Work out the finished part from the listing and answer in its coordinate system (mm). A direction names the side the tool comes from. Give positions to 0.01 mm unless a question says otherwise; leave off trailing zeros. One line per item, written item: value.
from build123d import *

# Parameters (mm, degrees)
F0_R     = 14
F1_DEPTH = 1.6
F2_R     = 2.25
F3_DEPTH = 2.2


with BuildPart() as f1:
    # F0 (on Top) → F1 (new body)
    with BuildSketch(Plane.XY):
        with BuildLine():
            Line((55.331106, 31.643028), (43.487067, 43.487067))
            Line((43.487067, 43.487067), (31.643028, 55.331106))
            ThreePointArc((31.643028, 55.331106), (16.240585, 49.856732), (0, 48))
            ThreePointArc((0, 48), (-16.240585, 49.856732), (-31.643028, 55.331106))
            Line((-31.643028, 55.331106), (-43.487067, 43.487067))
            Line((-43.487067, 43.487067), (-55.331106, 31.643028))
            ThreePointArc((-55.331106, 31.643028), (-49.856732, 16.240585), (-48, 0))
            ThreePointArc((-48, 0), (-49.856732, -16.240585), (-55.331106, -31.643028))
            Line((-55.331106, -31.643028), (-43.487067, -43.487067))
            Line((-43.487067, -43.487067), (-31.643028, -55.331106))
            ThreePointArc((-31.643028, -55.331106), (-16.240585, -49.856732), (0, -48))
            ThreePointArc((0, -48), (16.240585, -49.856732), (31.643028, -55.331106))
            Line((31.643028, -55.331106), (43.487067, -43.487067))
            Line((43.487067, -43.487067), (55.331106, -31.643028))
            ThreePointArc((55.331106, -31.643028), (49.856732, -16.240585), (48, 0))
            ThreePointArc((48, 0), (49.856732, 16.240585), (55.331106, 31.643028))
        make_face()
        with BuildLine():
            ThreePointArc((-40.092954, -40.092954), (-41.557421, -36.557421), (-40.092954, -33.021887))
            Line((-40.092954, -33.021887), (-32.385491, -25.314423))
            ThreePointArc((-32.385491, -25.314423), (-28.849957, -23.849957), (-25.314423, -25.314423))
            ThreePointArc((-25.314423, -25.314423), (-23.849957, -28.849957), (-25.314423, -32.385491))
            Line((-25.314423, -32.385491), (-33.021887, -40.092954))
            ThreePointArc((-33.021887, -40.092954), (-36.557421, -41.557421), (-40.092954, -40.092954))
        make_face(mode=Mode.SUBTRACT)
        with BuildLine():
            Line((8.8, -41.3), (0, -41.3))
            Line((0, -41.3), (-8.8, -41.3))
            ThreePointArc((-8.8, -41.3), (-11.3, -38.8), (-8.8, -36.3))
            Line((-8.8, -36.3), (0, -36.3))
            Line((0, -36.3), (8.8, -36.3))
            ThreePointArc((8.8, -36.3), (11.3, -38.8), (8.8, -41.3))
        make_face(mode=Mode.SUBTRACT)
        with BuildLine():
            ThreePointArc((0, -30.1), (1.8, -31.9), (0, -33.7))
            ThreePointArc((0, -33.7), (-1.8, -31.9), (0, -30.1))
        make_face(mode=Mode.SUBTRACT)
        with BuildLine():
            ThreePointArc((-18.596908, -18.596908), (-18.596908, -16.051324), (-16.051324, -16.051324))
            ThreePointArc((-16.051324, -16.051324), (-16.051324, -18.596908), (-18.596908, -18.596908))
        make_face(mode=Mode.SUBTRACT)
        with BuildLine():
            Line((6.6, -27.2), (0, -27.2))
            Line((0, -27.2), (-6.6, -27.2))
            ThreePointArc((-6.6, -27.2), (-11.3, -22.5), (-6.6, -17.8))
            Line((-6.6, -17.8), (0, -17.8))
            Line((0, -17.8), (6.6, -17.8))
            ThreePointArc((6.6, -17.8), (11.3, -22.5), (6.6, -27.2))
        make_face(mode=Mode.SUBTRACT)
        with BuildLine():
            ThreePointArc((25.314423, -25.314423), (28.849957, -23.849957), (32.385491, -25.314423))
            Line((32.385491, -25.314423), (40.092954, -33.021887))
            ThreePointArc((40.092954, -33.021887), (41.557421, -36.557421), (40.092954, -40.092954))
            ThreePointArc((40.092954, -40.092954), (36.557421, -41.557421), (33.021887, -40.092954))
            Line((33.021887, -40.092954), (25.314423, -32.385491))
            ThreePointArc((25.314423, -32.385491), (23.849957, -28.849957), (25.314423, -25.314423))
        make_face(mode=Mode.SUBTRACT)
        with BuildLine():
            ThreePointArc((18.596908, -18.596908), (16.051324, -18.596908), (16.051324, -16.051324))
            ThreePointArc((16.051324, -16.051324), (18.596908, -16.051324), (18.596908, -18.596908))
        make_face(mode=Mode.SUBTRACT)
        with BuildLine():
            Line((-36.3, 8.8), (-36.3, 0))
            Line((-36.3, 0), (-36.3, -8.8))
            ThreePointArc((-36.3, -8.8), (-38.8, -11.3), (-41.3, -8.8))
            Line((-41.3, -8.8), (-41.3, 0))
            Line((-41.3, 0), (-41.3, 8.8))
            ThreePointArc((-41.3, 8.8), (-38.8, 11.3), (-36.3, 8.8))
        make_face(mode=Mode.SUBTRACT)
        with BuildLine():
            ThreePointArc((-30.1, 0), (-31.9, -1.8), (-33.7, 0))
            ThreePointArc((-33.7, 0), (-31.9, 1.8), (-30.1, 0))
        make_face(mode=Mode.SUBTRACT)
        with BuildLine():
            ThreePointArc((-17.8, -6.6), (-22.5, -11.3), (-27.2, -6.6))
            Line((-27.2, -6.6), (-27.2, 0))
            Line((-27.2, 0), (-27.2, 6.6))
            ThreePointArc((-27.2, 6.6), (-22.5, 11.3), (-17.8, 6.6))
            Line((-17.8, 6.6), (-17.8, 0))
            Line((-17.8, 0), (-17.8, -6.6))
        make_face(mode=Mode.SUBTRACT)
        Circle(F0_R, mode=Mode.SUBTRACT)
        with BuildLine():
            ThreePointArc((-18.596908, 18.596908), (-16.051324, 18.596908), (-16.051324, 16.051324))
            ThreePointArc((-16.051324, 16.051324), (-18.596908, 16.051324), (-18.596908, 18.596908))
        make_face(mode=Mode.SUBTRACT)
        with BuildLine():
            Line((0, 27.2), (6.6, 27.2))
            ThreePointArc((6.6, 27.2), (11.3, 22.5), (6.6, 17.8))
            Line((6.6, 17.8), (0, 17.8))
            Line((0, 17.8), (-6.6, 17.8))
            ThreePointArc((-6.6, 17.8), (-11.3, 22.5), (-6.6, 27.2))
            Line((-6.6, 27.2), (0, 27.2))
        make_face(mode=Mode.SUBTRACT)
        with BuildLine():
            Line((-33.021887, 40.092954), (-25.314423, 32.385491))
            ThreePointArc((-25.314423, 32.385491), (-23.849957, 28.849957), (-25.314423, 25.314423))
            ThreePointArc((-25.314423, 25.314423), (-28.849957, 23.849957), (-32.385491, 25.314423))
            Line((-32.385491, 25.314423), (-40.092954, 33.021887))
            ThreePointArc((-40.092954, 33.021887), (-41.557421, 36.557421), (-40.092954, 40.092954))
            ThreePointArc((-40.092954, 40.092954), (-36.557421, 41.557421), (-33.021887, 40.092954))
        make_face(mode=Mode.SUBTRACT)
        with BuildLine():
            ThreePointArc((0, 30.1), (-1.8, 31.9), (0, 33.7))
            ThreePointArc((0, 33.7), (1.8, 31.9), (0, 30.1))
        make_face(mode=Mode.SUBTRACT)
        with BuildLine():
            Line((8.8, 36.3), (0, 36.3))
            Line((0, 36.3), (-8.8, 36.3))
            ThreePointArc((-8.8, 36.3), (-11.3, 38.8), (-8.8, 41.3))
            Line((-8.8, 41.3), (0, 41.3))
            Line((0, 41.3), (8.8, 41.3))
            ThreePointArc((8.8, 41.3), (11.3, 38.8), (8.8, 36.3))
        make_face(mode=Mode.SUBTRACT)
        with BuildLine():
            Line((17.8, -6.6), (17.8, 0))
            Line((17.8, 0), (17.8, 6.6))
            ThreePointArc((17.8, 6.6), (22.5, 11.3), (27.2, 6.6))
            Line((27.2, 6.6), (27.2, 0))
            Line((27.2, 0), (27.2, -6.6))
            ThreePointArc((27.2, -6.6), (22.5, -11.3), (17.8, -6.6))
        make_face(mode=Mode.SUBTRACT)
        with BuildLine():
            ThreePointArc((18.596908, 18.596908), (18.596908, 16.051324), (16.051324, 16.051324))
            ThreePointArc((16.051324, 16.051324), (16.051324, 18.596908), (18.596908, 18.596908))
        make_face(mode=Mode.SUBTRACT)
        with BuildLine():
            ThreePointArc((30.1, 0), (31.9, 1.8), (33.7, 0))
            ThreePointArc((33.7, 0), (31.9, -1.8), (30.1, 0))
        make_face(mode=Mode.SUBTRACT)
        with BuildLine():
            Line((36.3, -8.8), (36.3, 0))
            Line((36.3, 0), (36.3, 8.8))
            ThreePointArc((36.3, 8.8), (38.8, 11.3), (41.3, 8.8))
            Line((41.3, 8.8), (41.3, 0))
            Line((41.3, 0), (41.3, -8.8))
            ThreePointArc((41.3, -8.8), (38.8, -11.3), (36.3, -8.8))
        make_face(mode=Mode.SUBTRACT)
        with BuildLine():
            Line((40.092954, 33.021887), (32.385491, 25.314423))
            ThreePointArc((32.385491, 25.314423), (28.849957, 23.849957), (25.314423, 25.314423))
            ThreePointArc((25.314423, 25.314423), (23.849957, 28.849957), (25.314423, 32.385491))
            Line((25.314423, 32.385491), (33.021887, 40.092954))
            ThreePointArc((33.021887, 40.092954), (36.557421, 41.557421), (40.092954, 40.092954))
            ThreePointArc((40.092954, 40.092954), (41.557421, 36.557421), (40.092954, 33.021887))
        make_face(mode=Mode.SUBTRACT)
    extrude(amount=F1_DEPTH)

    # F2 (on face) → F3 (join)
    with BuildSketch(Plane.XY.offset(1.6)):
        with Locations((31.9, 19.95)):
            Circle(F2_R)
        with Locations((47.525639, 31.615736)):
            Circle(F2_R)
        with Locations((31.615736, 47.525639)):
            Circle(F2_R)
        with Locations((19.95, 31.9)):
            Circle(F2_R)
        with Locations((47.525639, -31.615736)):
            Circle(F2_R)
        with Locations((31.9, -19.95)):
            Circle(F2_R)
        with Locations((19.95, -31.9)):
            Circle(F2_R)
        with Locations((31.615736, -47.525639)):
            Circle(F2_R)
        with Locations((-31.9, -19.95)):
            Circle(F2_R)
        with Locations((-31.9, 19.95)):
            Circle(F2_R)
        with Locations((-47.525639, -31.615736)):
            Circle(F2_R)
        with Locations((-31.615736, 47.525639)):
            Circle(F2_R)
        with Locations((-47.525639, 31.615736)):
            Circle(F2_R)
        with Locations((-31.615736, -47.525639)):
            Circle(F2_R)
        with Locations((-19.95, 31.9)):
            Circle(F2_R)
        with Locations((-19.95, -31.9)):
            Circle(F2_R)
    extrude(amount=F3_DEPTH)


solid = f1.part
(1) Given P1, Ø2, axis at x = -10.5, y = -41, coming from the -Z side; P2, Ø4.5, axis at x = 17.32, y = 17.32, coming from the +Z side; P3, Ø1.3, axis at y = 0, z = 0.5, coming from the +X side; P4, Ø1, axis at y = 19, z = 2.5, coming from the -X side, each flat-ended and moving along its own axis, determine where each tip first touches the part or whether it passes through.
Findings:
P1: stops at z = 0
P2: stops at z = 1.6
P3: stops at x = 48
P4: stops at x = -34.1
(2) Find the intervals of material crossed by probe 1 along X at (y, z) = (-31.9, 1.1); probe 2 along X at (y, z) = (-7, 0.25), in increasing order. Write a range as from..to.
Findings:
probe 1: x = -55.07..-38.97, -24.89..-1.8, 1.8..24.89, 38.97..55.07
probe 2: x = -48.34..-41.3, -36.3..-27.18, -17.82..-12.12, 12.12..17.82, 27.18..36.3, 41.3..48.34
(3) Section A-A, the plane z = 2.55 is taken. Give the number of separate pieces and of enclosed holes in the cut face, then the cut area to 3 significant figures.
Findings:
separate pieces: 16
enclosed holes: 0
area: 254 mm^2
(4) Determine the mould class of faces 1 (the flat face through (43.653, 43.321, 0.789)), 2 (the flat face through (36.185, -29.114, 0.789)) for opening direction X: pulls with the +X half, pulls with the -X half, needs draft (parallel to the pull), parting line crosses it, or undercut.
Findings:
face 1: pulls with the +X half
face 2: undercut
(5) Which of the six approach directions +Z, -Z, +X, -X, +Y, -Y give full straight-line access (tool end or side, diameter ignored) to faces 3 (the flat face through (43.321, -43.653, 0.789)), 4 (the cylindrical face through (-38.9, 11.3, 0.8)), 5 (the cylindrical face through (-48.01, 29.42, 2.68))?
Findings:
face 3: +Z, -Z, +X, -Y
face 4: +Z, -Z
face 5: +Z
